Autodesk Inventor part; units mm, degrees
ref_plane "YZ Plane" through (0, 0, 0) normal (1, 0, 0) x (0, 1, 0)
ref_plane "XZ Plane" through (0, 0, 0) normal (0, 1, 0) x (-1, 0, 0)
ref_plane "XY Plane" through (0, 0, 0) normal (0, 0, 1) x (1, 0, 0)
sketch "Sketch1" plane through (0, 0, 0) normal (0, 1, 0) x (-1, 0, 0)
  line L0 (0, 0) -> (165.1, 0)
  line L1 (165.1, 0) -> (165.1, -203.2)
  line L2 (165.1, -203.2) -> (0, -203.2)
  line L3 (0, -203.2) -> (0, 0)
  line L4 (158.75, -196.85) -> (158.75, -6.35)
  line L5 (158.75, -6.35) -> (6.35, -6.35)
  line L6 (6.35, -6.35) -> (6.35, -196.85)
  line L7 (6.35, -196.85) -> (158.75, -196.85)
  line L8 (152.4, -190.5) -> (152.4, -12.7)
  line L9 (152.4, -12.7) -> (12.7, -12.7)
  line L10 (12.7, -12.7) -> (12.7, -190.5)
  line L11 (12.7, -190.5) -> (152.4, -190.5)
  dimension "d0" = 203.2
  dimension "d1" = 165.1
  dimension "d2" = 6.35
  dimension "d3" = 12.7
extrude "Extrusion1" add sketch "Sketch1" along normal blind 12.7 contours L0 L1 L2 L3 | L7 L6 L5 L4 | L11 L10 L9 L8
extrude "Extrusion2" add sketch "Sketch1" along normal blind 101.6 contours L0 L1 L2 L3
extrude "Extrusion3" add sketch "Sketch1" along normal blind 95.25 contours L7 L6 L5 L4
sketch "Sketch2" plane through (-165.1, 0, -203.2) normal (-1, 0, 0) x (0, 0, 1)
  line L0 (12.7, 12.7) -> (190.5, 12.7)
  line L1 (12.7, 28.575) -> (38.1, 28.575)
  line L2 (38.1, 28.575) -> (38.1, 3.175)
  line L3 (38.1, 3.175) -> (12.7, 3.175)
  line L4 (12.7, 3.175) -> (12.7, 28.575)
  line L5 (0, 0) -> (203.2, 0)
  dimension "d10" = 3.175
  dimension "d11" = 25.4
  dimension "d12" = 25.4
extrude "Extrusion4" cut sketch "Sketch2" against normal through all
properties part number "OGRobotBase" material "ABS Plastic"
The model under review builds one solid part; all positions refer to its coordinate system, in mm. A direction names the side the tool comes from. Coordinates: 2 decimals unless noted, no trailing zeros. Order: outer loops, then holes, each group sorted by start corner. A loop starts at its lowest first (then second) coordinate and runs counter-clockwise, first axis right, second up. Notation, with made-up numbers: (63.5, 14.5) -> (72.5, 14.5) arc R19 cw to (72.5, 34.5) -> close; hole circle Ø4 at (-38, 22.25). An arc over 180 degrees is marked (long way). Answer in a Markdown table with one row per item. Add a question column.
Item 1: We need section C-C on y = 39.5. Write out the cut boundary in (x, z).
Item 2: Machinability: for faces 4 (the flat face through (-84, 53, -12.7)), 5 (the flat face through (-81, 50, 0)), 6 (the flat face through (-159, 28.575, -178)), which of the approach directions +Z, -Z, +X, -X, +Y, -Y give a long, thin tool a straight path to every point of the face, cutting with its end or side? Answer none if there is none.
Item 3: Mouldability with a two-part tool opening along X and no side actions: class faces 1 (the flat face through (-9, 95.25, -101)), 2 (the flat face through (-6, 28.575, -178)), 3 (the flat face through (-165.1, 50, -100)) as +X half, -X half, draft (parallel to the pull), parting line (faces both ways), or undercut.
Item 4: We need section D-D on x = -65. Write out the cut boundary in (y, z) (3 decimals).
Item 5: We need section A-A on y = 24.5. Write out the cut boundary in (x, z).
Item 6: We need section B-B on z = -181.5. Write out the cut boundary in (x, y) (3 decimals), plus the area to 3 significant figures.
Item 7: To check wall thickness, follow probe 1 along X at (y, z) = (89.5, -40); probe 2 along Z at (x, y) = (-129.5, 67.5); probe 3 along Z at (x, y) = (-35, 8.5). State the ranges of each line that lie inside material, in increasing order.
Item 8: Clearance check with flat-ended pins moving along their axes: pin 1 (10 mm diameter, centred on x = -159.5, z = -179, fed in from -Y); pin 2 (3 mm diameter, centred on x = -121.5, z = -57.5, fed in from +Y). State where each tip first meets the part, or that it passes through.
Final values:
| question | item | result |
|---|---|---|
| 1 | outline | (-165.1, -203.2) -> (0, -203.2) -> (0, 0) -> (-165.1, 0) -> close; hole (-152.4, -190.5) -> (-12.7, -190.5) -> (-12.7, -12.7) -> (-152.4, -12.7) -> close |
| 2 | face 4 | +Y |
| 2 | face 5 | +Z, +X, -X, +Y, -Y |
| 2 | face 6 | +X, -X |
| 3 | face 1 | undercut |
| 3 | face 2 | draft |
| 3 | face 3 | -X half |
| 4 | outline | (0, -203.2) -> (101.6, -203.2) -> (101.6, -196.85) -> (95.25, -196.85) -> (95.25, -190.5) -> (3.175, -190.5) -> (3.175, -165.1) -> (12.7, -165.1) -> (12.7, -12.7) -> (95.25, -12.7) -> (95.25, -6.35) -> (101.6, -6.35) -> (101.6, 0) -> (0, 0) -> close |
| 5 | outline | (-165.1, -203.2) -> (0, -203.2) -> (0, -190.5) -> (-165.1, -190.5) -> close; (-165.1, -165.1) -> (-152.4, -165.1) -> (-152.4, -12.7) -> (-12.7, -12.7) -> (-12.7, -165.1) -> (0, -165.1) -> (0, 0) -> (-165.1, 0) -> close |
| 6 | outline | (-165.1, 0) -> (0, 0) -> (0, 3.175) -> (-165.1, 3.175) -> close; (-165.1, 28.575) -> (-152.4, 28.575) -> (-152.4, 95.25) -> (-158.75, 95.25) -> (-158.75, 101.6) -> (-165.1, 101.6) -> close; (-12.7, 28.575) -> (0, 28.575) -> (0, 101.6) -> (-6.35, 101.6) -> (-6.35, 95.25) -> (-12.7, 95.25) -> close |
| 6 | area | 2,300 mm2 |
| 7 | probe 1 | x = -165.1 to -152.4, -12.7 to 0 |
| 7 | probe 2 | z = -203.2 to -190.5, -12.7 to 0 |
| 7 | probe 3 | z = -203.2 to -190.5, -165.1 to 0 |
| 8 | pin 1 | stops at y = 0 |
| 8 | pin 2 | stops at y = 12.7 |
